from build123d import *

# Parameters (mm, degrees)
SKETCH_1_W                   = 120
SKETCH_1_H                   = 120
EXTRUDE_1_DEPTH              = 6
SKETCH_2_R                   = 3.5
CUT_EXTRUDE_1_DEPTH          = 10
FILLET_1_R                   = 10
HOLE_WIZARD_M3_1_D           = 3.4
HOLE_WIZARD_M3_1_CSINK_D     = 6.6
HOLE_WIZARD_M3_1_CSINK_ANGLE = 90
HOLE_WIZARD_M3_1_2_D         = 2.5
HOLE_WIZARD_M3_1_2_DEPTH     = 6
HOLE_WIZARD_M3_1_2_TIP       = 0.751075774


with BuildPart() as part:
    # 草图1 → 凸台-拉伸1 (new body)
    with BuildSketch(Plane(origin=(0, 0, 0), x_dir=(1, 0, 0), z_dir=(0, 1, 0))):
        Rectangle(SKETCH_1_W, SKETCH_1_H)
    extrude(amount=EXTRUDE_1_DEPTH)

    # 草图2 → 切除-拉伸1 (cut)
    with BuildSketch(Plane(origin=(0, 6, 0), x_dir=(1, 0, 0), z_dir=(0, 1, 0))):
        with Locations(Location((-50, 50, 0), (0, 0, 270))):
            Circle(SKETCH_2_R)
        with Locations(Location((50, 50, 0), (0, 0, 270))):
            Circle(SKETCH_2_R)
        with Locations(Location((50, -50, 0), (0, 0, 270))):
            Circle(SKETCH_2_R)
        with Locations(Location((-50, -50, 0), (0, 0, 270))):
            Circle(SKETCH_2_R)
    extrude(amount=-CUT_EXTRUDE_1_DEPTH, mode=Mode.SUBTRACT)

    # 圆角1
    fillet_1_edges = [part.edges().sort_by_distance(p)[0] for p in [
        (60, 3, 60),
        (-60, 3, 60),
        (-60, 3, -60),
        (60, 3, -60),
    ]]
    fillet(fillet_1_edges, radius=FILLET_1_R)

    # Hole Wizard M3 _1 (through all)
    with Locations(Plane.XZ):
        with Locations((15.969331282, -22.388176755), (22.388176755, -15.969331282), (22.388176755, 15.969331282), (15.969331282, 22.388176755), (-15.969331282, 22.388176755), (-22.388176755, 15.969331282), (-22.388176755, -15.969331282), (-15.969331282, -22.388176755)):
            CounterSinkHole(HOLE_WIZARD_M3_1_D / 2, HOLE_WIZARD_M3_1_CSINK_D / 2, counter_sink_angle=HOLE_WIZARD_M3_1_CSINK_ANGLE)

    # Hole Wizard M3 _1 2
    with Locations(Plane(origin=(0, 6, 0), x_dir=(1, 0, 0), z_dir=(0, 1, 0))):
        with Locations((-43, -10), (-43, 10), (43, -10), (43, 10)):
            Hole(HOLE_WIZARD_M3_1_2_D / 2, depth=HOLE_WIZARD_M3_1_2_DEPTH)
            with Locations((0, 0, -(HOLE_WIZARD_M3_1_2_DEPTH + HOLE_WIZARD_M3_1_2_TIP / 2))):  # 118° drill point
                Cone(0, HOLE_WIZARD_M3_1_2_D / 2, HOLE_WIZARD_M3_1_2_TIP, mode=Mode.SUBTRACT)


solid = part.part
Build history of the part. All positions in model axes, mm. Round coordinates to 2 decimals unless told otherwise and drop trailing zeros. Loops run counter-clockwise (first coordinate to the right, second up) from the corner with the lowest first, then second, coordinate; pieces in that order, holes last. Notation, with made-up numbers: (-34, 6.25) -> (-13, 6.25) arc R20 cw to (-13, 18.25) -> close; hole circle Ø6 at (9.25, 27.5). An arc over 180 degrees is marked (long way). Use CSV: the item, a comma, the result in double quotes. Start each with the question number.
Q1. Saw through at A-A on y = 4.3. Count the separate pieces of the cut face and the enclosed holes in it, and give its area (3 significant figures).
Q2. Saw through at B-B on x = 48. Give the cut face in (y, z), and give its area (3 significant figures).
Q3. Flat gauge pins, fed straight in: pin 1 Ø5.5 at (x, z) = (-15.97, 22.39) entering from -Y; pin 2 Ø12 at (x, z) = (44.5, 24) entering from -Y; pin 3 Ø4 at (x, z) = (-15.97, -22.39) entering from -Y. Where does each tip first touch, or does it go through?
Q4. Mould opens along X. For faces 1 (the face through (56.99, 3.04, 57.15)), 2 (the face through (-57.15, 3.04, 56.99)), 3 (the face through (-47.635, 3.042, -52.58)), 4 (the face through (15.185, 3.831, -23.896)) say: +X half, -X half, draft (parallel to the pull), parting line (faces both ways), or undercut.
Q5. Drill centre lines: L1, parallel to X at y = 2.25, z = 10; L2, parallel to Z at x = -42, y = 3.35; L3, parallel to X at y = 1.2, z = 11. Where is each one in solid material? Low to high.
Solutions:
1,separate pieces,"1"
1,enclosed holes,"16"
1,area,"14,100 mm^2"
2,outline,"(0, -60) -> (6, -60) -> (6, -52.87) -> (0, -52.87) -> close; (0, -47.13) -> (6, -47.13) -> (6, 47.13) -> (0, 47.13) -> close; (0, 52.87) -> (6, 52.87) -> (6, 60) -> (0, 60) -> close"
2,area,"651 mm^2"
3,pin 1,"stops at y = 0.55"
3,pin 2,"stops at y = 0"
3,pin 3,"stops at y = 1.3"
4,face 1,"+X half"
4,face 2,"-X half"
4,face 3,"undercut"
4,face 4,"undercut"
5,L1,"x = -60 to -44.25, -41.75 to 41.75, 44.25 to 60"
5,L2,"z = -60 to -10.75, -9.25 to 9.25, 10.75 to 60"
5,L3,"x = -60 to -43.75, -42.25 to 42.25, 43.75 to 60"
